CAD build for the part. Positions are in the model's coordinates, mm. A direction names the side the tool comes from. Give positions to 0.01 mm unless a question says otherwise; leave off trailing zeros. Loops run counter-clockwise (first coordinate to the right, second up) from the corner with the lowest first, then second, coordinate; pieces in that order, holes last. Notation, with made-up numbers: M 81.5,68.25 L 138.5,68.25 A29 ccw 138.5,102.25 Z; hole C 72.5,-11.5 d9. An arc over 180 degrees is marked long. Answer as CSV lines item,"result".
from build123d import *

# Parameters (mm, degrees)
F0_R      = 27.0383
F1_DEPTH  = 73.914
F2_R      = 24.13
F3_DEPTH  = 20.7264
F4_R      = 12.7
F5_DEPTH  = 2.54
F6_R      = 12.7
F6_R_2    = 4.699
F7_DEPTH  = 2.54
F8_R      = 3.175
F9_DEPTH  = 21.59
F10_R     = 6.731
F11_DEPTH = 34.925
F13_DEPTH = 6.35
F15_DEPTH = 12.7


with BuildPart() as f1:
    # F0 (on Top) → F1 (new body)
    with BuildSketch(Plane.XY):
        Circle(F0_R)
    extrude(amount=F1_DEPTH)

    # F2 (on face) → F3 (join)
    with BuildSketch(Plane.XY.offset(73.914)):
        Circle(F2_R)
    extrude(amount=F3_DEPTH)

    # F4 (on face) → F5 (join)
    with BuildSketch(Plane.XY.offset(94.6404)):
        Circle(F4_R)
    extrude(amount=F5_DEPTH)

    # F6 (on face) → F7 (join)
    with BuildSketch(Plane(origin=(0, 0, 0), x_dir=(1, 0, 0), z_dir=(0, 0, -1))):
        Circle(F6_R)
        Circle(F6_R_2, mode=Mode.SUBTRACT)
    extrude(amount=F7_DEPTH)

    # F8 (on face) → F9 (join)
    with BuildSketch(Plane(origin=(0, 0, 0), x_dir=(1, 0, 0), z_dir=(0, 0, -1))):
        Circle(F8_R)
    extrude(amount=F9_DEPTH)

    # F10 (on Front) → F11 (join, symmetric)
    with BuildSketch(Plane.XZ):
        with Locations((0, 80.772)):
            Circle(F10_R)
    extrude(amount=F11_DEPTH, both=True)

    # F12 (on face) → F13 (cut)
    with BuildSketch(Plane.XY.offset(94.6404)):
        with BuildLine():
            ThreePointArc((-15.8748731392, 10.00125), (-16.9479549257, 11.3997174113), (-18.5765047188, 10.72515))
            Line((-18.5765047188, 10.72515), (-16.0688415596, 9.27735))
            ThreePointArc((-16.0688415596, 9.27735), (-15.9242057279, 9.6265317865), (-15.8748731392, 10.00125))
        make_face()
        with BuildLine():
            Line((-16.0688415596, 9.27735), (-18.5765047188, 10.72515))
            ThreePointArc((-18.5765047188, 10.72515), (-18.0465731392, 8.7474184204), (-16.0688415596, 9.27735))
        make_face()
        with BuildLine():
            Line((0, -18.5547), (0, -21.4503))
            ThreePointArc((0, -21.4503), (1.0237491978, -21.0262491978), (1.4478, -20.0025))
            ThreePointArc((1.4478, -20.0025), (1.0237491978, -18.9787508022), (0, -18.5547))
        make_face()
        with BuildLine():
            ThreePointArc((0, -18.5547), (-1.4478, -20.0025), (0, -21.4503))
            Line((0, -21.4503), (0, -18.5547))
        make_face()
        with BuildLine():
            Line((16.0688415596, 9.27735), (18.5765047188, 10.72515))
            ThreePointArc((18.5765047188, 10.72515), (16.5987731392, 11.2550815796), (16.0688415596, 9.27735))
        make_face()
        with BuildLine():
            ThreePointArc((18.7704731392, 10.00125), (18.7211405505, 10.3759682135), (18.5765047188, 10.72515))
            Line((18.5765047188, 10.72515), (16.0688415596, 9.27735))
            ThreePointArc((16.0688415596, 9.27735), (17.6973913527, 8.6027825887), (18.7704731392, 10.00125))
        make_face()
    extrude(amount=-F13_DEPTH, mode=Mode.SUBTRACT)

    # F14 (on face) → F15 (cut)
    with BuildSketch(Plane(origin=(0, 0, 0), x_dir=(1, 0, 0), z_dir=(0, 0, -1))):
        with BuildLine():
            ThreePointArc((14.7363675327, 13.2666150431), (13.3965175327, 14.6064650431), (12.0566675327, 13.2666150431))
            Line((12.0566675327, 13.2666150431), (13.3965175327, 13.2666150431))
            Line((13.3965175327, 13.2666150431), (13.3965175327, 11.9267650431))
            ThreePointArc((13.3965175327, 11.9267650431), (14.3439345535, 12.3191980223), (14.7363675327, 13.2666150431))
        make_face()
        with BuildLine():
            Line((13.3965175327, 13.2666150431), (12.0566675327, 13.2666150431))
            ThreePointArc((12.0566675327, 13.2666150431), (12.4491005119, 12.3191980223), (13.3965175327, 11.9267650431))
            Line((13.3965175327, 11.9267650431), (13.3965175327, 13.2666150431))
        make_face()
        with BuildLine():
            ThreePointArc((14.7363675327, -13.6573849569), (14.3439345535, -12.7099679361), (13.3965175327, -12.3175349569))
            Line((13.3965175327, -12.3175349569), (13.3965175327, -13.6573849569))
            Line((13.3965175327, -13.6573849569), (12.0566675327, -13.6573849569))
            ThreePointArc((12.0566675327, -13.6573849569), (13.3965175327, -14.9972349569), (14.7363675327, -13.6573849569))
        make_face()
        with BuildLine():
            Line((13.3965175327, -13.6573849569), (13.3965175327, -12.3175349569))
            ThreePointArc((13.3965175327, -12.3175349569), (12.4491005119, -12.7099679361), (12.0566675327, -13.6573849569))
            Line((12.0566675327, -13.6573849569), (13.3965175327, -13.6573849569))
        make_face()
        with BuildLine():
            Line((-12.1812824673, 13.2666150431), (-13.5274824673, 13.2666150431))
            Line((-13.5274824673, 13.2666150431), (-13.5274824673, 11.9204150431))
            ThreePointArc((-13.5274824673, 11.9204150431), (-12.5755753185, 12.3147078943), (-12.1812824673, 13.2666150431))
        make_face()
        with BuildLine():
            Line((-13.5274824673, 11.9204150431), (-13.5274824673, 13.2666150431))
            Line((-13.5274824673, 13.2666150431), (-12.1812824673, 13.2666150431))
            ThreePointArc((-12.1812824673, 13.2666150431), (-14.4793896162, 14.2185221919), (-13.5274824673, 11.9204150431))
        make_face()
        with BuildLine():
            ThreePointArc((-12.1876324673, -13.6573849569), (-12.5800654465, -12.7099679361), (-13.5274824673, -12.3175349569))
            Line((-13.5274824673, -12.3175349569), (-13.5274824673, -13.6573849569))
            Line((-13.5274824673, -13.6573849569), (-12.1876324673, -13.6573849569))
        make_face()
        with BuildLine():
            Line((-13.5274824673, -13.6573849569), (-13.5274824673, -12.3175349569))
            ThreePointArc((-13.5274824673, -12.3175349569), (-14.4748994881, -14.6048019777), (-12.1876324673, -13.6573849569))
            Line((-12.1876324673, -13.6573849569), (-13.5274824673, -13.6573849569))
        make_face()
    extrude(amount=-F15_DEPTH, mode=Mode.SUBTRACT)


solid = f1.part
1) Band-saw the part on A-A on y = 0. Give the cut face in (x, z) (3 decimals), and give its area (3 significant figures).
Answer below:
outline,"M -27.038,0 L -12.7,0 L -12.7,-2.54 L -4.699,-2.54 L -4.699,0 L -3.175,0 L -3.175,-21.59 L 3.175,-21.59 L 3.175,0 L 4.699,0 L 4.699,-2.54 L 12.7,-2.54 L 12.7,0 L 27.038,0 L 27.038,73.914 L 24.13,73.914 L 24.13,94.64 L 12.7,94.64 L 12.7,97.18 L -12.7,97.18 L -12.7,94.64 L -24.13,94.64 L -24.13,73.914 L -27.038,73.914 Z"
area,"5,240 mm^2"
2) Which spindle directions (+Z, -Z, +X, -X, +Y, -Y) get a long thin tool onto all of the face, cutting with end or side? Do faces 5 (the face through (-6.724, 28.966, 81.068)), 6 (the face through (0, -20, 88.29)), 7 (the face through (-14, -13, 12.7)), 8 (the face through (0, -34.925, 81)), 9 (the face through (-0.876, -29.131, 87.446)). Say none if no direction does.
Answer below:
face 5,"+Y"
face 6,"+Z"
face 7,"-Z"
face 8,"+Z, -Z, +X, -X, -Y"
face 9,"-Y"
3) Flat gauge pins, fed straight in: pin 1 (3 mm diameter, centred on x = 13, y = 13, fed in from -Z); pin 2 (2.5 mm diameter, centred on x = 18, y = 10.5, fed in from +Z); pin 3 (1.5 mm diameter, centred on x = -19.5, z = 47.5, fed in from +Y). Where does each tip first touch, or does it go through?
Answer below:
pin 1,"stops at z = 0"
pin 2,"stops at z = 94.64"
pin 3,"stops at y = 19.48"
4) Drill centre lines: line 1 (X direction, y = 0, z = -0.45) (3 decimals); line 2 (Z direction, x = -17.5, y = -5); line 3 (Z direction, x = 4, y = -5.5). Where is each one in solid material? Low to high. Write a range as from..to.
Answer below:
line 1,"x = -12.7..-4.699, -3.175..3.175, 4.699..12.7"
line 2,"z = 0..94.64"
line 3,"z = -2.54..97.18"
5) Band-saw the part on B-B on x = 21.5. Give the cut face in (y, z), and give its area (3 significant figures).
Answer below:
outline,"M -16.4,0 L 16.4,0 L 16.4,73.91 L 10.95,73.91 L 10.95,94.64 L -10.95,94.64 L -10.95,73.91 L -16.4,73.91 Z"
area,"2,880 mm^2"
6) Band-saw the part on C-C on z = 70.5. Give the cut face in (x, y).
Answer below:
outline,"C 0,0 d54.08"
7) Band-saw the part on D-D on y = -8. Give the cut face in (x, z), and give its area (3 significant figures).
Answer below:
outline,"M -25.83,0 L -9.86,0 L -9.86,-2.54 L 9.86,-2.54 L 9.86,0 L 25.83,0 L 25.83,73.91 L 22.77,73.91 L 22.77,94.64 L 9.86,94.64 L 9.86,97.18 L -9.86,97.18 L -9.86,94.64 L -22.77,94.64 L -22.77,73.91 L -25.83,73.91 Z"
area,"4,860 mm^2"
8) Mould opens along Z. For faces 1 (the face through (-16.1, 18.2, 73.914)), 2 (the face through (6, -12, 0)), 3 (the face through (-0.61, -4.66, -1.25)), 4 (the face through (0, 0, 97.18)) say: +Z half, -Z half, draft (parallel to the pull), parting line (faces both ways), or undercut.
Answer below:
face 1,"undercut"
face 2,"-Z half"
face 3,"draft"
face 4,"+Z half"
